Here's how the part is built. I have some questions about the finished solid (model axes, mm). Face numbers are marked on the shaded views. A direction names the side the tool comes from. Round coordinates to 2 decimals unless told otherwise and drop trailing zeros. Order: outer loops, then holes, each group sorted by start corner. A loop starts at its lowest first (then second) coordinate and runs counter-clockwise, first axis right, second up. Notation, with made-up numbers: M 88.5,52 L 118.5,52 A19 cw 118.5,86 Z; hole C 15.5,-25.75 d10. An arc over 180 degrees is marked long. Answer as CSV lines item,"result". Start each with the question number.
Autodesk Fusion 360 part; units mm, degrees
sketch "Sketch1" plane through (0, 0, 0) normal (0, 0, 1) x (1, 0, 0)
  line L0 (7.1, 7.1) -> (-7.1, 7.1)
  line L1 (-7.1, 7.1) -> (-7.1, -7.1)
  line L2 (-7.1, -7.1) -> (7.1, -7.1)
  line L3 (7.1, -7.1) -> (7.1, 7.1)
  line L4 (0, 3) -> (0, -1) construction
  line L5 (-0.75, 3) -> (-0.75, -1)
  line L6 (0.75, 3) -> (0.75, -1)
  circle A0 centre (0, 3) radius 0.75
  line L7 (-3.0891, -3.6495) -> (0.375, -1.6495)
  circle A1 centre (-3.4641, -3) radius 0.75
  line L8 (-3.8391, -2.3505) -> (-0.375, -0.3505)
  line L9 (-3.4641, -3) -> (0, -1) construction
  line L10 (3.8391, -2.3505) -> (0.375, -0.3505)
  circle A2 centre (3.4641, -3) radius 0.75
  line L11 (3.0891, -3.6495) -> (-0.375, -1.6495)
  line L12 (3.4641, -3) -> (0, -1) construction
  line L13 (-4.2141, 3.75) -> (4.2141, 3.75)
  line L14 (4.2141, 3.75) -> (4.2141, -3.75)
  line L15 (4.2141, -3.75) -> (-4.2141, -3.75)
  line L16 (-4.2141, -3.75) -> (-4.2141, 3.75)
  line L17 (-7.1, 0) -> (7.1, 0) construction
  line L18 (0, 7.1) -> (0, -7.1) construction
  point P0 (0, -3.75)
  point P1 (-4.2141, 0)
  dimension "d38" = 14.2
  dimension "d41" = 4
  dimension "d42" = 0.75
  dimension "d43" = -0.75
  dimension "d45" = 360
extrude "Extrude1" add sketch "Sketch1" along normal blind 2 contours L0 L1 L2 L3 | L5 A0 A1 L8 L13 L16 | L6 A0 L10 A2 L13 L14 | A1 L15 L16 | A2 L14 L15 | L7 A1 A2 L11 L15
sketch "Sketch2" plane through (0, 0, 0) normal (0, 0, 1) x (1, 0, 0)
  line L0 (-33.9, 6.35) -> (-21.2, 6.35) construction
  line L1 (-21.2, 6.35) -> (-21.2, -6.35) construction
  line L2 (-21.2, -6.35) -> (-33.9, -6.35) construction
  line L3 (-33.9, -6.35) -> (-33.9, 6.35) construction
  line L4 (21.2, 6.35) -> (33.9, 6.35) construction
  line L5 (33.9, 6.35) -> (33.9, -6.35) construction
  line L6 (33.9, -6.35) -> (21.2, -6.35) construction
  line L7 (21.2, -6.35) -> (21.2, 6.35) construction
  line L8 (-21.2, 0) -> (21.2, 0) construction
  line L9 (-21.1, -6.45) -> (-34, -6.45)
  line L10 (-34, -6.45) -> (-34, 6.45)
  line L11 (-34, 6.45) -> (-21.1, 6.45)
  line L12 (-21.1, 6.45) -> (-21.1, -6.45)
  line L13 (-18.6, -8.95) -> (-36.5, -8.95)
  line L14 (-36.5, -8.95) -> (-36.5, 8.95)
  line L15 (-36.5, 8.95) -> (-18.6, 8.95)
  line L16 (-18.6, 8.95) -> (-18.6, -8.95)
  line L17 (0, 2.5) -> (0, 20)
  line L18 (34, -6.45) -> (34, 6.45)
  line L19 (34, 6.45) -> (21.1, 6.45)
  line L20 (21.1, 6.45) -> (21.1, -6.45)
  line L21 (21.1, -6.45) -> (34, -6.45)
  line L22 (36.5, -8.95) -> (36.5, 8.95)
  line L23 (36.5, 8.95) -> (18.6, 8.95)
  line L24 (18.6, -8.95) -> (36.5, -8.95)
  line L25 (18.6, 8.95) -> (18.6, -8.95)
  line L26 (-18.6, -2.6) -> (-18.6, -8.95)
  line L27 (-18.6, 8.95) -> (18.6, 8.95)
  line L28 (18.6, -8.95) -> (-18.6, -8.95)
  line L29 (-7.1, 7.1) -> (-7.1, -7.1)
  line L30 (-7.1, -7.1) -> (7.1, -7.1)
  line L31 (7.1, -7.1) -> (7.1, 7.1)
  line L32 (7.1, 7.1) -> (-7.1, 7.1)
  dimension "d18" = 12.7
  dimension "d19" = 12.7
  dimension "d20" = 42.4
  dimension "d23" = -2.5
extrude "Extrude2" add sketch "Sketch2" along normal blind 2
extrude "Extrude3" add sketch "Sketch2" against normal blind 19 contours L13 L14 L15 L16 L26 | L22 L23 L24 L25
fillet "Fillet1" radius 12 2 edges at (-18.6, 0, 0) (18.6, 0, 0)
sketch "Sketch3" plane through (0, 8.95, 0) normal (0, 1, 0) x (-1, 0, 0)
  line L0 (36.5, -19) -> (36.5, 2)
  line L1 (36.5, 2) -> (-36.5, 2)
  line L2 (18.6, -12) -> (18.6, -19)
  line L3 (-36.5, -19) -> (-18.6, -19)
  circle A0 centre (-27.55, -13.6) radius 2.075
  circle A1 centre (-27.55, -3.6) radius 2.075
  line L4 (-27.55, -19) -> (-27.55, 2) construction
  line L5 (-36.5, 2) -> (-36.5, -19)
  line L6 (-18.6, -19) -> (-18.6, -12)
  line L7 (18.6, -19) -> (36.5, -19)
  line L8 (0, 1.75) -> (0, 22.5)
  circle A2 centre (27.55, -13.6) radius 2.075
  circle A3 centre (27.55, -3.6) radius 2.075
  dimension "d32" = 4.15
  dimension "d33" = 10
  dimension "d34" = 5.6
extrude "Extrude4" cut sketch "Sketch3" against normal blind 17.9
sketch "Sketch4" plane through (0, 0, 2) normal (0, 0, 1) x (1, 0, 0)
  line L0 (36.5, -8.95) -> (36.5, 8.95)
  line L1 (36.5, 8.95) -> (-36.5, 8.95)
  line L2 (-36.5, 8.95) -> (-36.5, -8.95)
  line L3 (-36.5, -8.95) -> (36.5, -8.95)
  line L4 (-34, 6.45) -> (-21.1, 6.45)
  line L5 (-21.1, 6.45) -> (-21.1, -6.45)
  line L6 (-21.1, -6.45) -> (-34, -6.45)
  line L7 (-34, -6.45) -> (-34, 6.45)
  line L8 (34, -6.45) -> (21.1, -6.45)
  line L9 (21.1, -6.45) -> (21.1, 6.45)
  line L10 (21.1, 6.45) -> (34, 6.45)
  line L11 (34, 6.45) -> (34, -6.45)
  line L12 (0.75, -0.567) -> (3.8391, -2.3505)
  arc A0 (3.0891, -3.6495) -> (3.8391, -2.3505) centre (3.4641, -3) ccw
  line L13 (3.0891, -3.6495) -> (0, -1.866)
  line L14 (0, -1.866) -> (-3.0891, -3.6495)
  arc A1 (-3.8391, -2.3505) -> (-3.0891, -3.6495) centre (-3.4641, -3) ccw
  line L15 (-3.8391, -2.3505) -> (-0.75, -0.567)
  line L16 (-0.75, -0.567) -> (-0.75, 3)
  arc A2 (0.75, 3) -> (-0.75, 3) centre (0, 3) ccw
  line L17 (0.75, 3) -> (0.75, -0.567)
  line L18 (21.1, -6.45) -> (21.1, 6.45)
  line L19 (-21.1, 6.45) -> (-21.1, -6.45)
  circle A3 centre (-14.1, 0) radius 2.075
  line L20 (-21.1, 0) -> (21.1, 0) construction
  line L21 (0, 2.5) -> (0, 20)
  circle A4 centre (14.1, 0) radius 2.075
  dimension "d47" = 4.15
  dimension "d48" = 7
extrude "Extrude5" cut sketch "Sketch4" against normal blind 21 contours A3 | A4
ref_plane "WorkPlane1" through (0, 0, -8) normal (0, 0, -1) x (-1, 0, 0)
sketch "Sketch5" plane through (0, 0, -8) normal (0, 0, -1) x (-1, 0, 0)
  line L0 (-21.1, 6.45) -> (-21.1, -6.45)
  line L1 (21.1, -6.45) -> (21.1, 6.45)
  line L2 (-21.1, 0) -> (21.1, 0) construction
  circle A0 centre (-14.1, 0) radius 4.5
  line L3 (-17.7, 2.7) -> (-17.7, -2.7)
  line L4 (0, 1.75) -> (0, 22.5)
  circle A1 centre (14.1, 0) radius 4.5
  line L5 (17.7, 2.7) -> (17.7, -2.7)
  dimension "d52" = 9
  dimension "d53" = 7
  dimension "d54" = 3.6
extrude "Extrude6" cut sketch "Sketch5" against normal blind 8 contours A0 L3 | A1 L5 picked at (-15.0162, 0.2196) picked at (17.8896, -0.5649)
equation "mounting_size = 1.5 mm"
equation "d16 = frontal_width"
equation "tolerance_bar = 0.1 mm"
equation "d25 = frontal_width"
equation "d30 = 13 mm - ( 4 / 4 ) * 1 mm"
equation "tolerance_hole = 0.15 mm"
equation "d32 = 4 mm + tolerance_hole"
equation "d42 = mounting_size / 2"
equation "d43 = -d42"
equation "frontal_width = 2 mm"
equation "d47 = 4 mm + tolerance_hole"
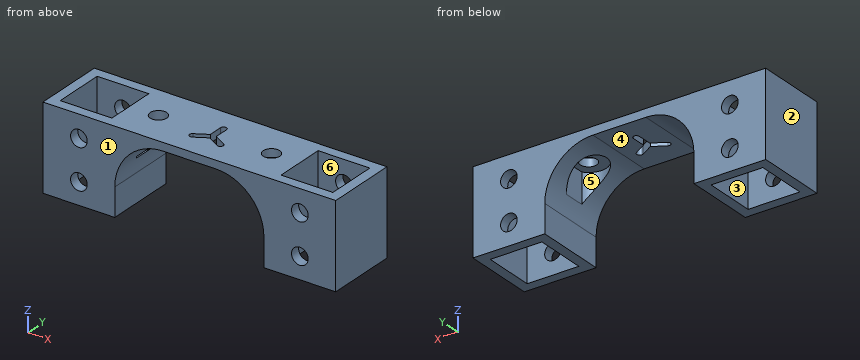
Item 1: If we section it at D-D on x = -27.55: Please give me the cut outline in (y, z) (3 decimals).
Item 2: Which directions (+Z, -Z, +X, -X, +Y, -Y) give clear straight access to the entire face, cutting with the end or side of a thin tool? Please do the marked faces 4, 5 and 6.
Item 3: If we section it at B-B on z = -13.6: Count the separate pieces of the cut face and the enclosed holes in it, and give its area (4 significant figures).
Item 4: If we section it at A-A on y = 5.5: Please give me the cut outline in (x, z), and give its area (3 significant figures).
Item 5: If we section it at C-C on x = 23: Please give me the cut outline in (y, z).
Item 6: For P1, Ø10, axis at x = -11.5, y = 0, coming from the -Z side; P2, Ø6.5, axis at x = -2.5, y = -4, coming from the -Z side, each with a flat end and sliding along its axis, tell me the tip position at first contact or that it passes through.
Item 7: If I drill on line 1 along Z through (x, y) = (-27.55, -7.4) (3 decimals); line 2 along X through (y, z) = (0, -4.5) (3 decimals); line 3 along Z through (x, y) = (-26, 7), over which ranges is the centre line in solid material (lowest first)?
Item 8: We'd pull the mould along Y, two halves only. Please class the marked faces 1, 2 and 3: pulls with the +Y half, pulls with the -Y half, needs draft (parallel to the pull), parting line crosses it, or undercut.
Geometry says:
1,outline,"M -8.95,-19 L -6.45,-19 L -6.45,-15.675 L -8.95,-15.675 Z; M -8.95,-11.525 L -6.45,-11.525 L -6.45,-5.675 L -8.95,-5.675 Z; M -8.95,-1.525 L -6.45,-1.525 L -6.45,2 L -8.95,2 Z; M 6.45,-19 L 8.95,-19 L 8.95,-15.675 L 6.45,-15.675 Z; M 6.45,-11.525 L 8.95,-11.525 L 8.95,-5.675 L 6.45,-5.675 Z; M 6.45,-1.525 L 8.95,-1.525 L 8.95,2 L 6.45,2 Z"
2,face 4,"-Z, +Y, -Y"
2,face 5,"-Z"
2,face 6,"+Z, -Z"
3,separate pieces,"4"
3,enclosed holes,"0"
3,area,"266.5 mm²"
4,outline,"M -36.5,-19 L -34,-19 L -34,2 L -36.5,2 Z; M -21.1,-19 L -18.6,-19 L -18.6,-12 A12 cw -6.6,0 L 6.6,0 A12 cw 18.6,-12 L 18.6,-19 L 21.1,-19 L 21.1,2 L -21.1,2 Z; M 34,-19 L 36.5,-19 L 36.5,2 L 34,2 Z"
4,area,"346 mm²"
5,outline,"M -8.95,-19 L -6.45,-19 L -6.45,2 L -8.95,2 Z; M 6.45,-19 L 8.95,-19 L 8.95,2 L 6.45,2 Z"
6,P1,"z = -5.22"
6,P2,"z = 0"
7,line 1,"-19 to -15.675, -11.525 to -5.675, -1.525 to 2"
7,line 2,"-36.5 to -34, -21.1 to -18.6, -17.7 to -16.175, 17.7 to 21.1, 34 to 36.5"
7,line 3,"-19 to -14.98, -12.22 to -4.98, -2.22 to 2"
8,face 1,"pulls with the -Y half"
8,face 2,"needs draft"
8,face 3,"undercut"
